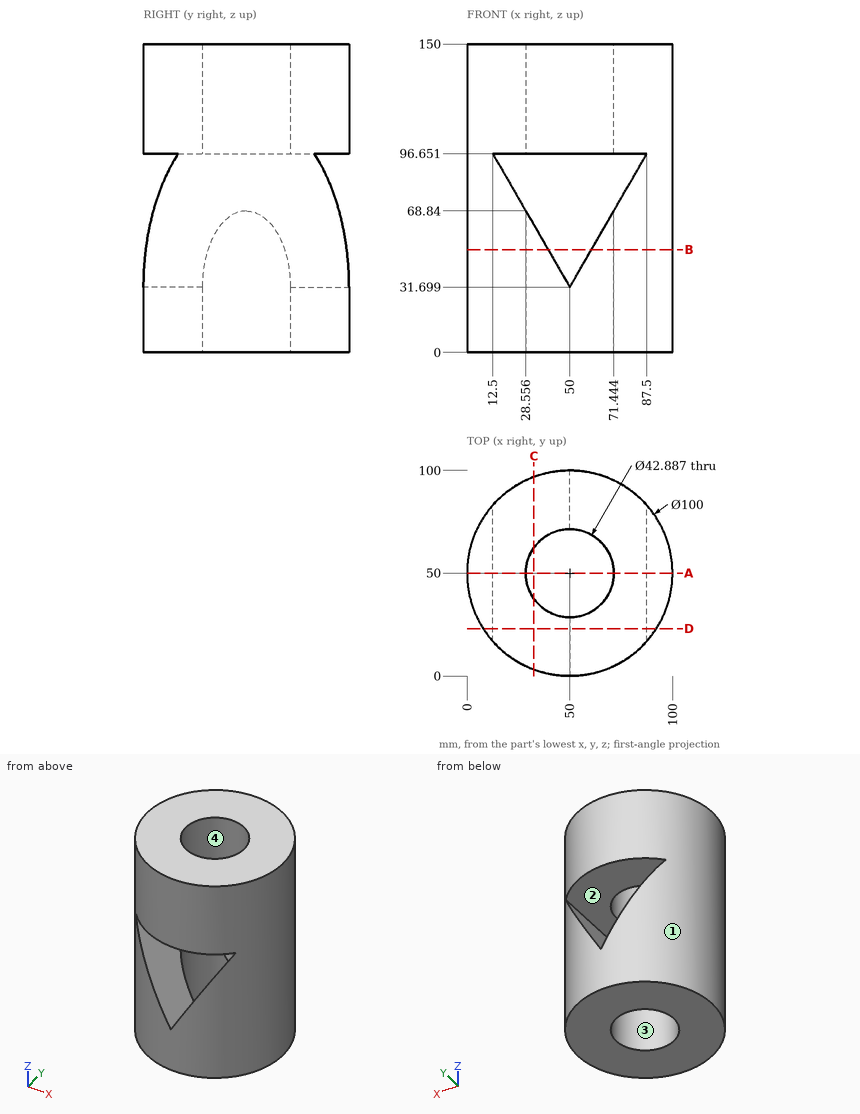
The figure shows three views and two pictorial views of one solid part (mm, origin at its lowest corner). Answer the questions. Give positions to 0.01 mm unless a question says otherwise; leave off trailing zeros. Write each loop counter-clockwise with the first axis right and the second up, starting at its lowest first coordinate (ties: lowest second). Pieces come first, ordered by that corner, then holes. Notation, with made-up numbers: (55.25, 6.25) - (84.25, 6.25) arc R16 cw to (84.25, 15.25) - close; hole circle Ø1 at (33, 65). An arc over 180 degrees is marked (long way). Use CSV: the item, a comma, the result in double quotes. Start each with the question number.
Item 1: The part is cut by section B-B, the plane z = 50. Give the vertices of the cut face in (x, y).
Item 2: The part is cut by section A-A, the plane y = 50. Give the vertices of the cut face in (x, z), and give its area (3 significant figures).
Item 3: Flat-ended cylindrical pins translate along their axes: P1, Ø5, axis at y = 61, z = 18.5, coming from the +X side; P2, Ø5, axis at x = 36.5, z = 36.5, coming from the +Y side (1 decimal); P3, Ø1.5, axis at x = 84, z = 118.5, coming from the +Y side. Find the tip coordinate at first contact, or state that the pin passes through.
Item 4: The part is cut by section C-C, the plane x = 32.5. Give the vertices of the cut face in (y, z).
Item 5: Consider line 1 (Y direction, x = 50, z = 17.5); line 2 (X direction, y = 35, z = 76.5) (1 decimal); line 3 (X direction, y = 71, z = 93) (1 decimal). Determine where each line is inside the solid, lowest interval first.
Item 6: The mould has two halves that part along Y. Classify the marked faces 1, 2, 3 and 4: pulls with the +Y half, pulls with the -Y half, needs draft (parallel to the pull), parting line crosses it, or undercut.
Item 7: The part is cut by section D-D, the plane y = 23. Give the vertices of the cut face in (x, z), and give its area (3 significant figures).
Taken from the geometry:
1,outline,"(39.43, 1.13) - (39.43, 31.34) arc R21.44 cw to (39.43, 68.66) - (39.43, 98.87) arc R50 ccw to start; (60.57, 1.13) arc R50 ccw to (60.57, 98.87) - (60.57, 68.66) arc R21.44 cw to (60.57, 31.34) - close"
2,outline,"(0, 0) - (28.56, 0) - (28.56, 68.84) - (12.5, 96.65) - (28.56, 96.65) - (28.56, 150) - (0, 150) - close; (71.44, 0) - (100, 0) - (100, 150) - (71.44, 150) - (71.44, 96.65) - (87.5, 96.65) - (71.44, 68.84) - close"
2,area,"8,120 mm2"
3,P1,"x = 99.27"
3,P2,"y = 98.8"
3,P3,"y = 87.34"
4,outline,"(3.16, 0) - (37.61, 0) - (37.61, 62.01) - (3.16, 62.01) - close; (3.16, 96.65) - (37.61, 96.65) - (37.61, 150) - (3.16, 150) - close; (62.39, 0) - (96.84, 0) - (96.84, 62.01) - (62.39, 62.01) - close; (62.39, 96.65) - (96.84, 96.65) - (96.84, 150) - (62.39, 150) - close"
5,line 1,"0 to 28.56, 71.44 to 100"
5,line 2,"2.3 to 24.1, 75.9 to 97.7"
5,line 3,"4.6 to 14.6, 85.4 to 95.4"
6,face 1,"parting line crosses it"
6,face 2,"needs draft"
6,face 3,"undercut"
6,face 4,"undercut"
7,outline,"(7.92, 0) - (92.08, 0) - (92.08, 150) - (7.92, 150) - close; hole (12.5, 96.65) - (50, 31.7) - (87.5, 96.65) - close"
7,area,"10,200 mm2"
